Input: part model. Units: mm. Frame: model coordinates. Face numbers are marked on the shaded views. A direction names the side the tool comes from. Round coordinates to 2 decimals unless told otherwise and drop trailing zeros. Order: outer loops, then holes, each group sorted by start corner. A loop starts at its lowest first (then second) coordinate and runs counter-clockwise, first axis right, second up. Notation, with made-up numbers: (-12.75, 17) -> (37.25, 17) arc R12 cw to (37.25, 30) -> close; hole circle Ø7 at (62, 20). An arc over 180 degrees is marked (long way). Use a Markdown table: item, result.
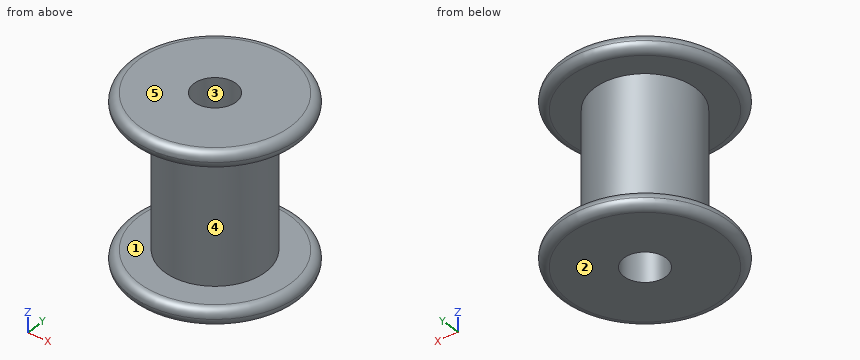
Autodesk Fusion 360 part; units mm, degrees
sketch "Esquisse1" plane through (0, 0, 0) normal (0, 0, 1) x (1, 0, 0)
  circle A0 centre (0, 0) radius 5
  dimension "d1" = 10
extrude "Extrusion1" add sketch "Esquisse1" along normal blind 1
sketch "Esquisse2" plane through (0, 0, 1) normal (0, 0, 1) x (-1, 0, 0)
  circle A0 centre (0, 0) radius 5
  circle A1 centre (0, 0) radius 3
  dimension "d4" = 6
extrude "Extrusion2" add sketch "Esquisse2" along normal blind 8 contours A1
sketch "Esquisse3" plane through (0, 0, 9) normal (0, 0, 1) x (-1, 0, 0)
  circle A0 centre (0, 0) radius 3
  circle A1 centre (0, 0) radius 5
  dimension "d7" = 10
extrude "Extrusion3" add sketch "Esquisse3" along normal blind 1 contours A0 | A1
sketch "Esquisse4" plane through (0, 0, 10) normal (0, 0, 1) x (-1, 0, 0)
  circle A0 centre (0, 0) radius 5
  circle A1 centre (0, 0) radius 1.25
  dimension "d10" = 2.5
extrude "Extrusion4" cut sketch "Esquisse4" against normal blind 10 contours A1
fillet "Congé1" radius 0.5 4 edges at (-4.6616, -1.8081, 1) (4.6616, 1.8081, 9) (4.6616, 1.8081, 10) (-4.6616, -1.8081, 0)
1) Cut plane C-C on z = 3.75. Return loops of the section in (x, y).
Results found:
| item | result |
|---|---|
| outline | circle Ø6 at (0, 0); hole circle Ø2.5 at (0, 0) |
2) Line query: L1, parallel to Z at x = -1.75, y = -3; L2, parallel to Y at x = 0, z = 3.25. Output: solid intervals per line, ascending. Write a range as [from, to].
Results found:
| item | result |
|---|---|
| L1 | z = [0, 1], [9, 10] |
| L2 | y = [-3, -1.25], [1.25, 3] |
3) Set-up query: the marked faces 4 and 5. Return all of +Z, -Z, +X, -X, +Y, -Y with unobstructed straight access to the full face (end or side cutting, diameter ignored); none if empty.
Results found:
| item | result |
|---|---|
| face 4 | none |
| face 5 | +Z, +X, -X, +Y, -Y |
4) Pin query (flat end, axial travel): pin 1 Ø4 at (y, z) = (-1, 6) entering from +X; pin 2 Ø5 at (x, z) = (-1, 4) entering from -Y; pin 3 Ø1.5 at (x, z) = (-2.5, 7.5) entering from -Y; pin 4 Ø3 at (x, y) = (0, 0) entering from +Z. Return the tip coordinate at first contact, or that it passes through.
Results found:
| item | result |
|---|---|
| pin 1 | stops at x = 3 |
| pin 2 | stops at y = -3 |
| pin 3 | stops at y = -2.44 |
| pin 4 | stops at z = 10 |
5) Pull-direction query (Z, two-part tool) for the marked faces 1, 2 and 3; classes: +Z half, -Z half, draft (parallel to the pull), parting line (faces both ways), or undercut.
Results found:
| item | result |
|---|---|
| face 1 | undercut |
| face 2 | -Z half |
| face 3 | draft |
